from build123d import *

# Parameters (mm, degrees)
SKETCH2_R           = 2.88
BOSS_EXTRUDE1_DEPTH = 0.250717968
SKETCH3_R           = 2.88
BOSS_EXTRUDE2_DEPTH = 0.069282032
BOSS_EXTRUDE2_TAPER = -60.000000004
SKETCH4_R           = 3
BOSS_EXTRUDE3_DEPTH = 19.68
SKETCH5_R           = 1.5705
BOSS_EXTRUDE4_DEPTH = 0.875
SKETCH6_R           = 1.5705
BOSS_EXTRUDE5_DEPTH = 0.4295
BOSS_EXTRUDE5_TAPER = -45
SKETCH7_R           = 2
BOSS_EXTRUDE6_DEPTH = 5.6955
CUT_EXTRUDE1_DEPTH  = 2
CHAMFER1_SIZE       = 0.4295
FILLET1_R           = 0.195


with BuildPart() as part:
    # Sketch1 → Revolve1 (revolve)
    with BuildSketch(Plane(origin=(0, 0, 0), x_dir=(-1, 0, 0), z_dir=(0, 0, -1))):
        with BuildLine():
            Line((0, 4.5), (0, 0))
            Line((0, 0), (4, 0))
            Line((4, 0), (4, 4.5))
            Line((4, 4.5), (2.2, 4.5))
            ThreePointArc((2.2, 4.5), (2, 4.3), (1.8, 4.5))
            Line((1.8, 4.5), (0, 4.5))
        make_face()
    revolve(axis=Axis((0, 0, 0), (-1, 0, 0)))

    # Sketch2 → Boss-Extrude1 (add)
    with BuildSketch(Plane(origin=(0, 0, 0), x_dir=(0, 0, -1), z_dir=(1, 0, 0))):
        Circle(SKETCH2_R)
    extrude(amount=BOSS_EXTRUDE1_DEPTH)

    # Sketch3 → Boss-Extrude2 (add)
    with BuildSketch(Plane(origin=(0.250717968, 0, 0), x_dir=(0, 0, -1), z_dir=(1, 0, 0))):
        Circle(SKETCH3_R)
    extrude(amount=BOSS_EXTRUDE2_DEPTH, taper=BOSS_EXTRUDE2_TAPER)

    # Sketch4 → Boss-Extrude3 (add)
    with BuildSketch(Plane(origin=(0.32, 0, 0), x_dir=(0, 0, -1), z_dir=(1, 0, 0))):
        Circle(SKETCH4_R)
    extrude(amount=BOSS_EXTRUDE3_DEPTH)

    # Sketch5 → Boss-Extrude4 (add)
    with BuildSketch(Plane(origin=(20, 0, 0), x_dir=(0, 0, -1), z_dir=(1, 0, 0))):
        Circle(SKETCH5_R)
    extrude(amount=BOSS_EXTRUDE4_DEPTH)

    # Sketch6 → Boss-Extrude5 (add)
    with BuildSketch(Plane(origin=(20.875, 0, 0), x_dir=(0, 0, -1), z_dir=(1, 0, 0))):
        Circle(SKETCH6_R)
    extrude(amount=BOSS_EXTRUDE5_DEPTH, taper=BOSS_EXTRUDE5_TAPER)

    # Sketch7 → Boss-Extrude6 (add)
    with BuildSketch(Plane(origin=(21.3045, 0, 0), x_dir=(0, 0, -1), z_dir=(1, 0, 0))):
        Circle(SKETCH7_R)
    extrude(amount=BOSS_EXTRUDE6_DEPTH)

    # Sketch8 → Cut-Extrude1 (cut)
    with BuildSketch(Plane.ZY.offset(4)):
        Polygon((1.5, -0.866025404), (1.5, 0.866025404), (0, 1.732050808), (-1.5, 0.866025404), (-1.5, -0.866025404), (0, -1.732050808), align=None)
    extrude(amount=-CUT_EXTRUDE1_DEPTH, mode=Mode.SUBTRACT)

    # Sketch9 → Cut-Revolve1 (revolve, cut)
    with BuildSketch(Plane.XY):
        Polygon((-2, 1.44), (-2, 0), (-1.168615612, 0), align=None)
    revolve(axis=Axis((-2, 0, 0), (1, 0, 0)), mode=Mode.SUBTRACT)

    # Chamfer1
    chamfer1_edges = [part.edges().sort_by_distance(p)[0] for p in [
        (27, 0, 2),
        (-4, -4.5, 0),
    ]]
    chamfer(chamfer1_edges, length=CHAMFER1_SIZE)

    # Fillet1
    fillet1_edges = [part.edges().sort_by_distance(p)[0] for p in [
        (0, 0, 2.88),
    ]]
    fillet(fillet1_edges, radius=FILLET1_R)


solid = part.part
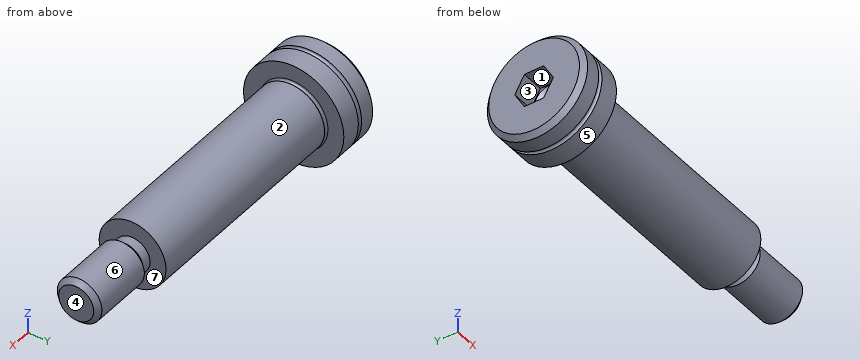
Part model, mm, in its own coordinate system. Face numbers are marked on the shaded views. A direction names the side the tool comes from. Coordinates: 2 decimals unless noted, no trailing zeros. Loops run counter-clockwise (first coordinate to the right, second up) from the corner with the lowest first, then second, coordinate; pieces in that order, holes last. Notation, with made-up numbers: (4, 55) -> (25, 55) arc R20 ccw to (25, 61) -> close; hole circle Ø8 at (75, 46). An arc over 180 degrees is marked (long way). Use a Markdown table: item, result. Add a question column.
Item 1: Band-saw the part on B-B on x = -1.5. Write the cut outline in (y, z), plus the area to 3 significant figures.
Item 2: Which spindle directions (+Z, -Z, +X, -X, +Y, -Y) get a long thin tool onto all of the face, cutting with end or side? Do the marked faces 5, 6 and 7. Say none if no direction does.
Item 3: Pull direction Y, two halves, no side cores. Call the marked faces 1, 2, 3 and 4: +Y half, -Y half, draft (parallel to the pull), parting line (faces both ways), or undercut.
Item 4: Band-saw the part on A-A on x = 14. Write the cut outline in (y, z).
Item 5: Probe probe 1 along X at (y, z) = (0.5, 2.5); probe 2 along X at (y, z) = (-1.5, -0.25); probe 3 along Y at (x, z) = (-0.5, -0.25). List the from-to ranges inside material, lowest first.
Item 6: Flat gauge pins, fed straight in: P1, Ø2, axis at y = -3, z = -1, coming from the +X side; P2, Ø4, axis at x = -1, y = -2.5, coming from the +Z side; P3, Ø1, axis at x = 5.5, y = -1.5, coming from the +Z side. Where does each tip first touch, or does it go through?
Geometry says:
| question | item | result |
|---|---|---|
| 1 | outline | circle Ø9 at (0, 0); hole circle Ø1.15 at (0, 0) |
| 1 | area | 62.6 mm² |
| 2 | face 5 | +X, -X |
| 2 | face 6 | +X |
| 2 | face 7 | none |
| 3 | face 1 | undercut |
| 3 | face 2 | parting line |
| 3 | face 3 | undercut |
| 3 | face 4 | draft |
| 4 | outline | circle Ø6 at (0, 0) |
| 5 | probe 1 | -4 to 20 |
| 5 | probe 2 | -2 to 27 |
| 5 | probe 3 | -4.49 to 4.49 |
| 6 | P1 | x = 20 |
| 6 | P2 | z = 4.47 |
| 6 | P3 | z = 2.83 |
